from build123d import *

# Parameters (mm, degrees)
CROQUIS1_R              = 37.5
SALIENTE_EXTRUIR1_DEPTH = 5
CROQUIS2_R              = 25
CROQUIS2_R_2            = 7.9375
SALIENTE_EXTRUIR2_DEPTH = 20
CROQUIS3_R              = 3.175
CORTAR_EXTRUIR2_DEPTH   = 65


with BuildPart() as part:
    # Croquis1 → Saliente-Extruir1 (new body)
    with BuildSketch(Plane.XY):
        with BuildLine():
            Line((-5, 0), (-40, 0))
            ThreePointArc((-40, 0), (-47.071067812, 2.928932188), (-50, 10))
            Line((-50, 10), (-50, 90))
            ThreePointArc((-50, 90), (-47.071067812, 97.071067812), (-40, 100))
            Line((-40, 100), (40, 100))
            ThreePointArc((40, 100), (47.071067812, 97.071067812), (50, 90))
            Line((50, 90), (50, -90))
            ThreePointArc((50, -90), (47.071067812, -97.071067812), (40, -100))
            Line((40, -100), (10, -100))
            ThreePointArc((10, -100), (2.928932188, -97.071067812), (0, -90))
            Line((0, -90), (0, -5))
            ThreePointArc((0, -5), (-1.464466094, -1.464466094), (-5, 0))
        make_face()
        with Locations((0, 50)):
            Circle(CROQUIS1_R, mode=Mode.SUBTRACT)
    extrude(amount=SALIENTE_EXTRUIR1_DEPTH)

    # Croquis2 → Saliente-Extruir2 (add)
    with BuildSketch(Plane(origin=(0, 0, 0), x_dir=(-1, 0, 0), z_dir=(0, 0, -1))):
        with Locations((-25, -75)):
            Circle(CROQUIS2_R)
        with Locations((-25, -75)):
            Circle(CROQUIS2_R_2, mode=Mode.SUBTRACT)
    extrude(amount=-SALIENTE_EXTRUIR2_DEPTH)

    # Croquis3 → Cortar-Extruir2 (cut)
    with BuildSketch(Plane(origin=(0, 0, 0), x_dir=(0, 0, -1), z_dir=(1, 0, 0))):
        with Locations((10, -75)):
            Circle(CROQUIS3_R)
        with Locations(Location((-15, -75, 0), (0, 0, 180))):
            Circle(CROQUIS3_R)
    extrude(amount=CORTAR_EXTRUIR2_DEPTH, mode=Mode.SUBTRACT)


solid = part.part
Build history of the part. All positions in model axes, mm. A direction names the side the tool comes from. Give positions to 0.01 mm unless a question says otherwise; leave off trailing zeros. Loops run counter-clockwise (first coordinate to the right, second up) from the corner with the lowest first, then second, coordinate; pieces in that order, holes last. Notation, with made-up numbers: (-10.5, 70.5) - (35.5, 70.5) arc R26 cw to (35.5, 96.5) - close; hole circle Ø8 at (83.5, 76). An arc over 180 degrees is marked (long way). Write item = value, one per line. Start each with the question number.
1) Band-saw the part on B-B on x = 6.5. Count the separate pieces of the cut face and the enclosed holes in it, plus the area to 3 significant figures.
2) Tool access for faces 1 (the cylindrical face through (46.99, 97.15, 2.46)), 2 (the cylindrical face through (1.154, -67.491, 12.395)), 3 (the flat face through (-22, 0, 2)): list every direction of +Z, -Z, +X, -X, +Y, -Y with a clear straight run to the whole face (end or side of a thin tool).
3) Probe probe 1 along Z at (x, y) = (9, -75) (3 decimals); probe 2 along Y at (x, z) = (25, 10); probe 3 along Z at (x, y) = (12, 13). List the from-to ranges inside material, lowest first. Write a range as from..to.
4) Band-saw the part on D-D on x = 30. Give the cut face in (y, z), plus the area to 3 significant figures.
5) Pull direction X, two halves, no side cores. Call faces 4 (the cylindrical face through (-8.13, 13.39, 2.46)), 5 (the flat face through (44, -94, 5)), 6 (the flat face through (0, -48, 2)): +X half, -X half, draft (parallel to the pull), parting line (faces both ways), or undercut.
6) Band-saw the part on C-C on z = 15. Give the cut face in (x, y) (1 decimal), plus the area to 3 significant figures.
7) Drop flat-ended pins along their axis: pin 1 Ø5 at (y, z) = (-53, 9) entering from +X; pin 2 Ø1 at (y, z) = (-79, 10.5) entering from +X; pin 3 Ø1.5 at (x, z) = (-31, 3) entering from -Y. Give the stop position or say it passes through.
8) Band-saw the part on A-A on y = 50. Give the cut face in (x, z).
Final values:
q1.separate_pieces = 2
q1.enclosed_holes = 1
q1.area = 1,100 mm²
q2.face_1 = +Z, -Z, +X, +Y
q2.face_2 = +Z
q2.face_3 = +Z, -Z, -X, -Y
q3.probe_1 = 0..11.825, 18.175..20
q3.probe_2 = -100..-82.94, -67.06..-50
q3.probe_3 = 0..5
q4.outline = (-100, 0) - (27.5, 0) - (27.5, 5) - (-50.51, 5) - (-50.51, 20) - (-68.84, 20) - (-68.84, 5) - (-81.16, 5) - (-81.16, 20) - (-99.49, 20) - (-99.49, 5) - (-100, 5) - close; (72.5, 0) - (100, 0) - (100, 5) - (72.5, 5) - close
q4.area = 1,320 mm²
q5.face_4 = undercut
q5.face_5 = draft
q5.face_6 = -X half
q6.outline = (0.2, -78.2) arc R25 ccw to (49.8, -78.2) - (32.3, -78.2) arc R7.9 cw to (17.7, -78.2) - close; (0.2, -71.8) - (17.7, -71.8) arc R7.9 cw to (32.3, -71.8) - (49.8, -71.8) arc R25 ccw to start
q6.area = 1,550 mm²
q7.pin_1 = 40.64
q7.pin_2 = 49.75
q7.pin_3 = 0
q8.outline = (-50, 0) - (-37.5, 0) - (-37.5, 5) - (-50, 5) - close; (37.5, 0) - (50, 0) - (50, 5) - (37.5, 5) - close
